Work out the finished part from the listing and answer in its coordinate system (mm). A direction names the side the tool comes from. Coordinates: 2 decimals unless noted, no trailing zeros. Order: outer loops, then holes, each group sorted by start corner. A loop starts at its lowest first (then second) coordinate and runs counter-clockwise, first axis right, second up.
1. The part is cut by section B-B, the plane x = 1090. Give the vertices of the cut face in (y, z) (3 decimals).
2. The part is cut by section D-D, the plane y = 145.5. Give the vertices of the cut face in (x, z), then the cut area to 3 significant figures.
3. Flat-ended cylindrical pins translate along their axes: pin 1 Ø5.5 at (x, y) = (1090, 12) entering from +Z; pin 2 Ø2 at (x, y) = (1087.5, 89.5) entering from +Z. Find the tip coordinate at first contact, or state that the pin passes through.
4. The part is cut by section C-C, the plane y = 12. Give the vertices of the cut face in (x, z), then the cut area to 3 significant figures.
5. A tool of negligible diameter and unlimited length cuts with its end or side. For faces 1 (the flat face through (1088, 101, 0.75)), 2 (the flat face through (1095, 86, 0)), from which of +Z, -Z, +X, -X, +Y, -Y can it reach the whole face along a straight path? Write none if from no direction.
6. Find the intervals of material crossed by probe 1 along Y at (x, z) = (1090, 2.3) (3 decimals); probe 2 along X at (y, z) = (159.5, 1.45); probe 3 along Y at (x, z) = (1090, -0.05) (3 decimals), in increasing order.
7. Determine the mould class of faces 3 (the cylindrical face through (1091.518, 158.532, -0.771)), 4 (the flat face through (1090, 0, 0)), 5 (the flat face through (1090, 169, 0)) for opening direction Y: +Y half, -Y half, draft (parallel to the pull), parting line (faces both ways), or undercut.
8. The part is cut by section A-A, the plane z = 1.7. Give the vertices of the cut face in (x, y) (3 decimals), then the cut area to 3 significant figures.
```python
from build123d import *

# Parameters (mm, degrees)
EXTRUDE_1_DEPTH              = 169
HOLE_WIZARD_M3_1_D           = 3.6
HOLE_WIZARD_M3_1_DEPTH       = 5
HOLE_WIZARD_M3_1_CBORE_D     = 7
HOLE_WIZARD_M3_1_CBORE_DEPTH = 2


with BuildPart() as part:
    # 草图1 → 凸台-拉伸1 (new body)
    with BuildSketch(Plane(origin=(0, 169, 0), x_dir=(1, 0, 0), z_dir=(0, 1, 0))):
        with BuildLine():
            Line((1095, -2.499371855), (1095, 2.25))
            Line((1095, 2.25), (1085, 2.25))
            Line((1085, 2.25), (1085, -2.499371855))
            ThreePointArc((1085, -2.499371855), (1090, -2.75), (1095, -2.499371855))
        make_face()
    extrude(amount=-EXTRUDE_1_DEPTH)

    # M3 六角头机械螺钉的柱形沉头孔1
    with Locations(Plane(origin=(1090, 101.825, 2.75), x_dir=(0, 1, 0), z_dir=(0, 0, 1))):
        with Locations((0, 0)):
            CounterBoreHole(HOLE_WIZARD_M3_1_D / 2, HOLE_WIZARD_M3_1_CBORE_D / 2, HOLE_WIZARD_M3_1_CBORE_DEPTH, depth=HOLE_WIZARD_M3_1_DEPTH)

    # 草图4 → 切除-旋转1 (revolve, cut)
    with BuildSketch(Plane(origin=(1090, 0, 0), x_dir=(0, 0, -1), z_dir=(1, 0, 0))):
        Polygon((-2.75, 159.5), (-2.75, 156), (-0.75, 156), (-0.75, 157.7), (2.25, 157.7), (2.25, 159.5), align=None)
    revolve(axis=Axis((1090, 159.5, -2.25), (0, 0, 1)), mode=Mode.SUBTRACT)

    # 草图5 → 切除-旋转2 (revolve, cut)
    with BuildSketch(Plane(origin=(1090, 0, 0), x_dir=(0, 0, -1), z_dir=(1, 0, 0))):
        Polygon((-2.75, 12), (-2.75, 8.5), (-0.75, 8.5), (-0.75, 10.2), (2.25, 10.2), (2.25, 12), align=None)
    revolve(axis=Axis((1090, 12, 2.75), (0, 0, -1)), mode=Mode.SUBTRACT)


solid = part.part
```
Geometry says:
1. outline: (0, -2.25) - (10.2, -2.25) - (10.2, 0.75) - (8.5, 0.75) - (8.5, 2.75) - (0, 2.75) - close; (13.8, -2.25) - (100.025, -2.25) - (100.025, 0.75) - (98.325, 0.75) - (98.325, 2.75) - (15.5, 2.75) - (15.5, 0.75) - (13.8, 0.75) - close; (103.625, -2.25) - (157.7, -2.25) - (157.7, 0.75) - (156, 0.75) - (156, 2.75) - (105.325, 2.75) - (105.325, 0.75) - (103.625, 0.75) - close; (161.3, -2.25) - (169, -2.25) - (169, 2.75) - (163, 2.75) - (163, 0.75) - (161.3, 0.75) - close
2. outline: (1085, -2.25) - (1095, -2.25) - (1095, 2.5) arc R50 ccw to (1085, 2.5) - close
2. area: 49.2 mm2
3. pin 1: stops at z = 0.75
3. pin 2: stops at z = 2.73
4. outline: (1085, -2.25) - (1088.2, -2.25) - (1088.2, 0.75) - (1086.5, 0.75) - (1086.5, 2.63) arc R50 ccw to (1085, 2.5) - close; (1091.8, -2.25) - (1095, -2.25) - (1095, 2.5) arc R50 ccw to (1093.5, 2.63) - (1093.5, 0.75) - (1091.8, 0.75) - close
4. area: 24.7 mm2
5. face 1: +Z
5. face 2: +Z, -Z, +X, +Y, -Y
6. probe 1: y = 0 to 8.5, 15.5 to 98.325, 105.325 to 156, 163 to 169
6. probe 2: x = 1085 to 1086.5, 1093.5 to 1095
6. probe 3: y = 0 to 10.2, 13.8 to 100.025, 103.625 to 157.7, 161.3 to 169
7. face 3: undercut
7. face 4: -Y half
7. face 5: +Y half
8. outline: (1085, 0) - (1095, 0) - (1095, 169) - (1085, 169) - close; hole circle Ø7 at (1090, 12); hole circle Ø7 at (1090, 101.825); hole circle Ø7 at (1090, 159.5)
8. area: 1,570 mm2
